Input: part model. Units: mm. Frame: model coordinates. A direction names the side the tool comes from. Coordinates: 2 decimals unless noted, no trailing zeros. Write each loop counter-clockwise with the first axis right and the second up, starting at its lowest first coordinate (ties: lowest second). Pieces come first, ordered by that corner, then holes. Notation, with made-up numbers: M 30,71 L 70,71 A30 cw 70,104 Z; hole C 11,82.5 d3. An arc over 180 degrees is marked long. Answer as a JSON object with one key per item and string values. Group by question number.
Autodesk Inventor part; units mm, degrees
ref_plane "YZ Plane" through (0, 0, 0) normal (1, 0, 0) x (0, 1, 0)
ref_plane "XZ Plane" through (0, 0, 0) normal (0, 1, 0) x (-1, 0, 0)
ref_plane "XY Plane" through (0, 0, 0) normal (0, 0, 1) x (1, 0, 0)
sketch "Sketch1" plane through (0, 0, 0) normal (0, 1, 0) x (-1, 0, 0)
  line L0 (0, -16.7083) -> (-14.4698, -8.3542)
  line L1 (-14.4698, -8.3542) -> (-14.4698, 8.3542)
  line L2 (-14.4698, 8.3542) -> (0, 16.7083)
  line L3 (0, 16.7083) -> (14.4698, 8.3542)
  line L4 (14.4698, 8.3542) -> (14.4698, -8.3542)
  line L5 (14.4698, -8.3542) -> (0, -16.7083)
  circle A0 centre (0, 0) radius 5
  dimension "d0" = 10
extrude "Extrusion1" add sketch "Sketch1" along normal blind 20
thread "Thread1"
sketch "Sketch2" plane through (0, 20, 0) normal (0, 1, 0) x (1, 0, 0)
  circle A0 centre (-10, 0) radius 2
  circle A1 centre (0, 10) radius 2
  circle A2 centre (0, -10) radius 2
  circle A3 centre (10, 0) radius 2
  point P0 (0, 0)
  dimension "d6" = 4
  dimension "d7" = 4
  dimension "d8" = 4
  dimension "d9" = 4
extrude "Extrusion2" add sketch "Sketch2" along normal blind 5
properties part number "Nut"
Q1. Section C-C, the plane y = 2.25. Return the cut outline in (x, z), and give its area (3 significant figures).
Q2. Section B-B, the plane x = 3.25. Return the cut outline in (y, z).
Q3. Section A-A, the plane z = 0. Return the cut outline in (x, y), and give its area (3 significant figures).
Q4. Line query: line 1 (Z direction, x = 0, y = 13.5); line 2 (Y direction, x = -3.5, z = -10); line 3 (Z direction, x = 2.25, y = 9). Output: solid intervals per line, ascending. Write a range as from..to.
Q5. Access query for faces 1 (the flat face through (10, 25, 0)), 2 (the cylindrical face through (-11.6, 22.5, -1.2)). Directions: +Z, -Z, +X, -X, +Y, -Y. A direction counts if a zero-diameter tool reaches every point of the face in a straight line with its end or side. Return the directions, or none.
Q6. Pin query (flat end, axial travel): pin 1 Ø1 at (x, y) = (8.5, 13) entering from -Z; pin 2 Ø1.5 at (x, y) = (-11, 11.5) entering from -Z; pin 3 Ø5 at (x, y) = (-5, 12.5) entering from -Z; pin 4 Ø6 at (x, z) = (0, 0) entering from +Y. Return the tip coordinate at first contact, or that it passes through.
Q7. Section D-D, the plane y = 22.25. Return the cut outline in (x, z), and give its area (3 significant figures).
Q8. Draft query along Z for faces 3 (the cylindrical face through (0, 22, -8)), 4 (the cylindrical face through (0, 22, 12)), 5 (the flat face through (7.13, 9.86, -12.59)), 6 (the cylindrical face through (8.4, 22.5, -1.2)). Return one class per face: released by +Z, released by -Z, zero draft, split by the parting line, or undercut.
Filled in:
{
 "1": {"outline": "M -14.47,-8.35 L 0,-16.71 L 14.47,-8.35 L 14.47,8.35 L 0,16.71 L -14.47,8.35 Z; hole C 0,0 d10", "area": "647 mm^2"},
 "2": {"outline": "M 0,-14.83 L 20,-14.83 L 20,-3.8 L 0,-3.8 Z; M 0,3.8 L 20,3.8 L 20,14.83 L 0,14.83 Z"},
 "3": {"outline": "M -14.47,0 L -5,0 L -5,20 L -8,20 L -8,25 L -12,25 L -12,20 L -14.47,20 Z; M 5,0 L 14.47,0 L 14.47,20 L 12,20 L 12,25 L 8,25 L 8,20 L 5,20 Z", "area": "419 mm^2"},
 "4": {"line 1": "-16.71..-5, 5..16.71", "line 2": "0..20", "line 3": "-15.41..-4.47, 4.47..15.41"},
 "5": {"face 1": "+Z, -Z, +X, -X, +Y", "face 2": "+Y"},
 "6": {"pin 1": "z = -12.09", "pin 2": "z = -10.79", "pin 3": "z = -15.26", "pin 4": "through"},
 "7": {"outline": "C -10,0 d4; C 0,-10 d4; C 0,10 d4; C 10,0 d4", "area": "50.3 mm^2"},
 "8": {"face 3": "undercut", "face 4": "undercut", "face 5": "released by -Z", "face 6": "split by the parting line"}
}
